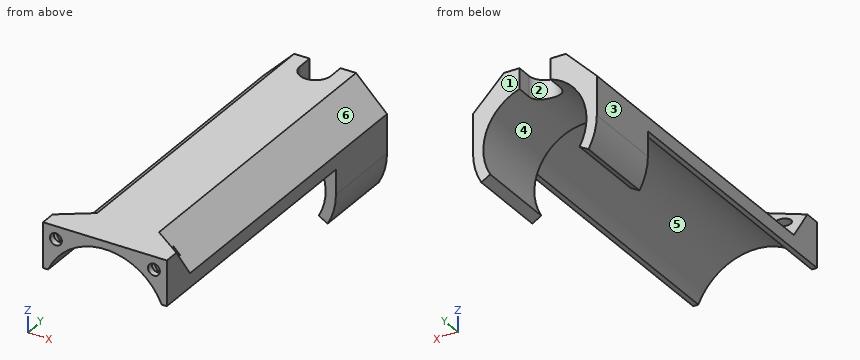
from build123d import *

# Parameters (mm, degrees)
BOSS_EXTRUDE1_DEPTH      = 56
BOSS_EXTRUDE2_DEPTH      = 16
BOSS_EXTRUDE3_DEPTH      = 3
BOSS_EXTRUDE3_DEPTH_BACK = 8
SKETCH4_W                = 24
SKETCH4_H                = 27
SKETCH5_W                = 28.405044576
SKETCH5_H                = 3.736732925
CUT_EXTRUDE2_DEPTH       = 78.826730626
CUT_EXTRUDE3_DEPTH       = 75.231058305
CUT_EXTRUDE5_DEPTH       = 3
CUT_EXTRUDE5_DEPTH_BACK  = 75.231058305
SKETCH8_W                = 24
SKETCH8_H                = 27
BOSS_EXTRUDE4_DEPTH      = 3
CHAMFER1_SIZE            = 4.25
SKETCH14_R               = 1.15
CUT_EXTRUDE8_DEPTH       = 8
CUT_EXTRUDE9_START       = -3
CUT_EXTRUDE9_DEPTH       = 1.8


with BuildPart() as part:
    # Sketch2 → Boss-Extrude1 (new body)
    with BuildSketch(Plane(origin=(0, 0, 0), x_dir=(1, 0, 0), z_dir=(0, 1, 0))):
        with BuildLine():
            Line((12, -13.5), (-12, -13.5))
            Line((-12, -13.5), (-12, -4.795831523))
            Line((-12, -4.795831523), (-11, -4.795831523))
            ThreePointArc((-11, -4.795831523), (0, -12), (11, -4.795831523))
            Line((11, -4.795831523), (12, -4.795831523))
            Line((12, -4.795831523), (12, -13.5))
        make_face()
    extrude(amount=BOSS_EXTRUDE1_DEPTH)

    # Sketch3 → Boss-Extrude2 (add)
    with BuildSketch(Plane(origin=(0, 56, 0), x_dir=(1, 0, 0), z_dir=(0, 1, 0))):
        with BuildLine():
            Line((-12, -13.5), (12, -13.5))
            Line((12, -13.5), (12, 0))
            ThreePointArc((12, 0), (11.591109915, 3.105828541), (10.392304845, 6))
            Line((10.392304845, 6), (8.660254038, 5))
            ThreePointArc((8.660254038, 5), (0, -10), (-8.660254038, 5))
            Line((-8.660254038, 5), (-10.392304845, 6))
            ThreePointArc((-10.392304845, 6), (-11.591109915, 3.105828541), (-12, 0))
            Line((-12, 0), (-12, -13.5))
        make_face()
    extrude(amount=BOSS_EXTRUDE2_DEPTH)

    # Sketch4 → Boss-Extrude3 (add, two sides: drawn at the far end of the back side and taken through both)
    with BuildSketch(Plane(origin=(0, 0, 0), x_dir=(1, 0, 0), z_dir=(0, 1, 0)).offset(-BOSS_EXTRUDE3_DEPTH_BACK)):
        Rectangle(SKETCH4_W, SKETCH4_H)
    extrude(amount=BOSS_EXTRUDE3_DEPTH + BOSS_EXTRUDE3_DEPTH_BACK)

    # Sketch5 → Cut-Revolve1 (revolve, cut)
    with BuildSketch(Plane(origin=(0, 0, 0), x_dir=(0, 0, -1), z_dir=(1, 0, 0))):
        with Locations((0.702522288, -8.868366462)):
            Rectangle(SKETCH5_W, SKETCH5_H)
    revolve(axis=Axis((0, 72, 13.5), (0, 0, -1)), mode=Mode.SUBTRACT)

    # Sketch6 → Cut-Extrude2 (cut, through all)
    with BuildSketch(Plane.XY.offset(13.5)):
        with BuildLine():
            Line((-3, 72), (-3, 69))
            ThreePointArc((-3, 69), (0, 66), (3, 69))
            Line((3, 69), (3, 72))
            Line((3, 72), (-3, 72))
        make_face()
    extrude(amount=-CUT_EXTRUDE2_DEPTH, mode=Mode.SUBTRACT)

    # Sketch7 → Cut-Extrude3 (cut, through all)
    with BuildSketch(Plane(origin=(0, 0, 0), x_dir=(1, 0, 0), z_dir=(0, 1, 0))):
        Polygon((6, -13.5), (12, -7.5), (12, -13.5), align=None)
        Polygon((-6, -13.5), (-12, -13.5), (-12, -7.5), align=None)
    extrude(amount=CUT_EXTRUDE3_DEPTH, mode=Mode.SUBTRACT)

    # Sketch8 → Cut-Extrude5 (cut, two sides: drawn at the far end of the back side and taken through both)
    with BuildSketch(Plane(origin=(0, 0, 0), x_dir=(1, 0, 0), z_dir=(0, 1, 0)).offset(-CUT_EXTRUDE5_DEPTH_BACK)):
        Rectangle(SKETCH8_W, SKETCH8_H)
    extrude(amount=CUT_EXTRUDE5_DEPTH + CUT_EXTRUDE5_DEPTH_BACK, mode=Mode.SUBTRACT)

    # Sketch13 → Boss-Extrude4 (add)
    with BuildSketch(Plane.XZ.offset(-3)):
        Polygon((-12, 7.5), (-12, 13.5), (-6, 13.5), align=None)
        Polygon((6, 13.5), (12, 13.5), (12, 7.5), align=None)
    extrude(amount=-BOSS_EXTRUDE4_DEPTH)

    # Chamfer1
    # the kernel refuses this chamfer: 4.25 mm, written as the material it adds along each edge
    with BuildSketch(Plane(origin=(1.728431539, 6, 21.228431539), x_dir=(-0.7068394360706696, -0.02749587661058644, 0.7068394360706773), z_dir=(-0.7071067811865515, 0, -0.7071067811865437))) as chamfer1_piece_1_section:
        Polygon((CHAMFER1_SIZE * 0.999621916911, CHAMFER1_SIZE * 0.0274958766106), (-CHAMFER1_SIZE * 0.0274958766106, CHAMFER1_SIZE * 0.999621916911), (0, 0), align=None)
    chamfer1_piece_1 = extrude(amount=30.344586772, mode=Mode.PRIVATE)
    chamfer1_piece_1 = split(chamfer1_piece_1, bisect_by=Plane(origin=(-12, 7.617398018, 11.205698206), z_dir=(1, 0, 0)), keep=Keep.TOP, mode=Mode.PRIVATE)
    chamfer1_piece_1 = split(chamfer1_piece_1, bisect_by=Plane(origin=(-9.705698206, 7.617398018, 13.5), z_dir=(0, 0, -1)), keep=Keep.TOP, mode=Mode.PRIVATE)
    add(chamfer1_piece_1)
    with BuildSketch(Plane(origin=(19.728431539, 6, -0.228431539), x_dir=(0.70683943607067, -0.02749587661058643, 0.706839436070677), z_dir=(-0.707106781186551, 0, 0.7071067811865441))) as chamfer1_piece_2_section:
        Polygon((CHAMFER1_SIZE * 0.999621916911, CHAMFER1_SIZE * 0.0274958766106), (-CHAMFER1_SIZE * 0.0274958766106, CHAMFER1_SIZE * 0.999621916911), (0, 0), align=None)
    chamfer1_piece_2 = extrude(amount=30.344586772, mode=Mode.PRIVATE)
    chamfer1_piece_2 = split(chamfer1_piece_2, bisect_by=Plane(origin=(12, 7.617398018, 11.205698206), z_dir=(-1, 0, 0)), keep=Keep.TOP, mode=Mode.PRIVATE)
    chamfer1_piece_2 = split(chamfer1_piece_2, bisect_by=Plane(origin=(9.705698206, 7.617398018, 13.5), z_dir=(0, 0, -1)), keep=Keep.TOP, mode=Mode.PRIVATE)
    add(chamfer1_piece_2)

    # Sketch14 → Cut-Extrude8 (cut)
    with BuildSketch(Plane.XZ.offset(-3)):
        with Locations(Location((-9.5, 11, 0), (0, 0, 270))):
            Circle(SKETCH14_R)
        with Locations(Location((9.5, 11, 0), (0, 0, 277.057128313))):
            Circle(SKETCH14_R)
    extrude(amount=-CUT_EXTRUDE8_DEPTH, mode=Mode.SUBTRACT)

    # Sketch15 → Cut-Extrude9 (cut)
    with BuildSketch(Plane.XZ.offset(-3).offset(CUT_EXTRUDE9_START)):
        Polygon((-7.190598923, 11), (-8.345299462, 13), (-10.654700538, 13), (-11.809401077, 11), (-10.654700538, 9), (-8.345299462, 9), align=None)
        Polygon((11.809401077, 11), (10.654700538, 13), (8.345299462, 13), (7.190598923, 11), (8.345299462, 9), (10.654700538, 9), align=None)
    extrude(amount=CUT_EXTRUDE9_DEPTH, mode=Mode.SUBTRACT)


solid = part.part
Could you check a few things on this model? Use its own coordinates, in mm. Face numbers are marked on the shaded views. A direction names the side the tool comes from. Round coordinates to 2 decimals unless told otherwise and drop trailing zeros. Write each loop counter-clockwise with the first axis right and the second up, starting at its lowest first coordinate (ties: lowest second). Pieces come first, ordered by that corner, then holes. Notation, with made-up numbers: (8, 28) - (58, 28) arc R22 ccw to (58, 34) - close; hole circle Ø6 at (30.5, -9.75). An arc over 180 degrees is marked (long way). Use a Markdown table: item, result.
Q1. For pin 1 (8 mm diameter, centred on x = 5, y = 54.5, fed in from -Z); pin 2 (1.1 mm diameter, centred on x = -11.5, y = 39.5, fed in from -Z); pin 3 (0.5 mm diameter, centred on x = 9, y = 5, fed in from -Z), each with a flat end and sliding along its axis, tell me the tip position at first contact or that it passes through.
Output values:
| item | result |
|---|---|
| pin 1 | z = -5.03 |
| pin 2 | z = 4.8 |
| pin 3 | z = 7.64 |
Q2. I want a section at D-D (z = -1.75). List the corners of the cut face in (x, y) for me.
Output values:
| item | result |
|---|---|
| outline | (-11.87, 56) - (-9.85, 56) - (-9.85, 72) - (-11.87, 72) - close; (9.85, 56) - (11.87, 56) - (11.87, 72) - (9.85, 72) - close |
Q3. I want a section at B-B (z = 3.5). List the corners of the cut face in (x, y) for me.
Output values:
| item | result |
|---|---|
| outline | (-12, 56) - (-9.37, 56) - (-9.37, 72) - (-12, 72) - close; (9.37, 56) - (12, 56) - (12, 72) - (9.37, 72) - close |
Q4. For the marked faces 4, 5 and 6, which set-ups out of +Z, -Z, +X, -X, +Y, -Y let a thin tool reach every point of the face, with its end or its side?
Output values:
| item | result |
|---|---|
| face 4 | +Y, -Y |
| face 5 | -Z, -Y |
| face 6 | +Z, +X, +Y |
Q5. I want a section at A-A (y = 55). List the corners of the cut face in (x, z) for me, plus the area to 3 significant figures.
Output values:
| item | result |
|---|---|
| outline | (-12, 4.8) - (-11, 4.8) arc R12 cw to (11, 4.8) - (12, 4.8) - (12, 7.5) - (6, 13.5) - (-6, 13.5) - (-12, 7.5) - close |
| area | 58.7 mm2 |
Q6. Please list where these lines run through material, in increasing order: L1, parallel to X at y = 3.75, z = 11; L2, parallel to X at y = 61.75, z = 0; L3, parallel to Z at x = 0, y = 60.5.
Output values:
| item | result |
|---|---|
| L1 | -12 to -10.65, -8.35 to -4.8, 4.8 to 8.35, 10.65 to 12 |
| L2 | -12 to -10, 10 to 12 |
| L3 | 10 to 13.5 |
Q7. Thinking about a two-plate mould opening in X: for the marked faces 1, 2 and 3, which applies, released by +X, released by -X, zero draft, split by the parting line, or undercut?
Output values:
| item | result |
|---|---|
| face 1 | zero draft |
| face 2 | undercut |
| face 3 | released by -X |
Q8. I want a section at C-C (x = 0). List the corners of the cut face in (y, z) for me.
Output values:
| item | result |
|---|---|
| outline | (3, 12) - (56, 12) - (56, 10) - (66, 10) - (66, 13.5) - (3, 13.5) - close |
